Build history of the part. All positions in model axes, mm. A direction names the side the tool comes from. Give positions to 0.01 mm unless a question says otherwise; leave off trailing zeros. Write each loop counter-clockwise with the first axis right and the second up, starting at its lowest first coordinate (ties: lowest second). Pieces come first, ordered by that corner, then holes. Notation, with made-up numbers: M 68.25,64.25 L 84.25,64.25 A27 ccw 84.25,86.25 Z; hole C -5,15 d9. An arc over 180 degrees is marked long. Return JSON: item names as keys, results as strings. Group by question number.
Q1. Tool access for faces 4 (the flat face through (49, 1, 12.7)), 5 (the flat face through (74, 2, -18.694)), 6 (the flat face through (31.14, 2, -15)): list every direction of +Z, -Z, +X, -X, +Y, -Y with a clear straight run to the whole face (end or side of a thin tool).
Q2. Pull direction X, two halves, no side cores. Call faces 1 (the flat face through (-80.721, 2, 0)), 2 (the flat face through (0, 1, 12.7)), 3 (the flat face through (25, 2, -18.694)): +X half, -X half, draft (parallel to the pull), parting line (faces both ways), or undercut.
Q3. Band-saw the part on A-A, the plane x = 2.5. Give the cut face in (y, z).
Q4. Flat gauge pins, fed straight in: pin 1 Ø1.5 at (x, y) = (-55.5, 1.5) entering from -Z; pin 2 Ø0.9 at (x, y) = (-5, 1.5) entering from +Z. Where does each tip first touch, or does it go through?
Q5. Wall check: probe 1 along X at (y, z) = (2.85, 13.5); probe 2 along Z at (x, y) = (-66.5, 0.85). Give the ranges that are in metal, low to high.
from build123d import *

# Parameters (mm, degrees)
SKETCH1_W            = 161.4424
SKETCH1_H            = 25.4
BOSS_EXTRUDE1_DEPTH  = 2.9972
SKETCH2_W            = 12.7
SKETCH2_H            = 5.9944
BOSS_EXTRUDE2_DEPTH  = 2.9972
FILLET1_R            = 1.778
FILLET1_OF_MIRROR1_R = 1.778


with BuildPart() as part:
    # Sketch1 → Boss-Extrude1 (new body)
    with BuildSketch(Plane(origin=(0, 0, 0), x_dir=(1, 0, 0), z_dir=(0, 1, 0))):
        Rectangle(SKETCH1_W, SKETCH1_H)
    extrude(amount=BOSS_EXTRUDE1_DEPTH)

    # Sketch2 → Boss-Extrude2 (add)
    with BuildSketch(Plane(origin=(0, 2.9972, 0), x_dir=(1, 0, 0), z_dir=(0, 1, 0))):
        with Locations((-74.3712, 15.6972)):
            Rectangle(SKETCH2_W, SKETCH2_H)
        with Locations((-24.7904, 15.6972)):
            Rectangle(SKETCH2_W, SKETCH2_H)
        with Locations((24.7904, 15.6972)):
            Rectangle(SKETCH2_W, SKETCH2_H)
        with Locations((74.3712, 15.6972)):
            Rectangle(SKETCH2_W, SKETCH2_H)
    boss_extrude2 = extrude(amount=-BOSS_EXTRUDE2_DEPTH)

    # Fillet1
    fillet1_edges = [part.edges().sort_by_distance(p)[0] for p in [
        (-68.0212, 1.4986, -18.6944),
        (-80.7212, 1.4986, -18.6944),
        (-18.4404, 1.4986, -18.6944),
        (-31.1404, 1.4986, -18.6944),
        (31.1404, 1.4986, -18.6944),
        (18.4404, 1.4986, -18.6944),
        (68.0212, 1.4986, -18.6944),
        (80.7212, 1.4986, -18.6944),
    ]]
    fillet(fillet1_edges, radius=FILLET1_R)

    # Mirror1: Boss-Extrude2 across plane
    add(boss_extrude2.mirror(Plane.XY))

    # Fillet1 of Mirror1
    fillet1_of_mirror1_edges = [part.edges().sort_by_distance(p)[0] for p in [
        (-68.0212, 1.4986, 18.6944),
        (-80.7212, 1.4986, 18.6944),
        (-18.4404, 1.4986, 18.6944),
        (-31.1404, 1.4986, 18.6944),
        (31.1404, 1.4986, 18.6944),
        (18.4404, 1.4986, 18.6944),
        (68.0212, 1.4986, 18.6944),
        (80.7212, 1.4986, 18.6944),
    ]]
    fillet(fillet1_of_mirror1_edges, radius=FILLET1_OF_MIRROR1_R)


solid = part.part
From the geometry:
{
 "1": {"face 4": "+Z, +Y, -Y", "face 5": "-Z, +X, -X, +Y, -Y", "face 6": "-Z, +Y, -Y"},
 "2": {"face 1": "-X half", "face 2": "undercut", "face 3": "draft"},
 "3": {"outline": "M 0,-12.7 L 3,-12.7 L 3,12.7 L 0,12.7 Z"},
 "4": {"pin 1": "stops at z = -12.7", "pin 2": "stops at z = 12.7"},
 "5": {"probe 1": "x = -80.72 to -68.02, -31.14 to -18.44, 18.44 to 31.14, 68.02 to 80.72", "probe 2": "z = -12.7 to 12.7"}
}
